Geometry check sheet. Reference: the model listing, model coordinates, mm. Face numbers are marked on the shaded views. Give positions to 0.01 mm unless a question says otherwise; leave off trailing zeros. Loops run counter-clockwise (first coordinate to the right, second up) from the corner with the lowest first, then second, coordinate; pieces in that order, holes last. Notation, with made-up numbers: (0, -38.75) -> (53, -38.75) arc R18 cw to (53, -29.75) -> close; hole circle Ø10 at (7.5, 47). An arc over 180 degrees is marked (long way). One line per question, with ' | ' between items.
from build123d import *

# Parameters (mm, degrees)
F0_R        = 45
F1_DEPTH    = 5
F2_R        = 36
F2_R_2      = 33.5
F3_DEPTH    = 70
F5_DEPTH    = 65
F6_R        = 3.4
F7_DEPTH    = 5.001
F8_T2_ANGLE = 64.3663587264
F8_T4_ANGLE = 60.259047326
F9_SIZE     = 5


# Not quite as in the source:
# - a fillet or chamfer that OpenCascade refuses, or shapes differently, is made with other operations: its cross-section is extruded or revolved along the edge and cut away or added


with BuildPart() as f1:
    # F0 (on Top) → F1 (new body)
    with BuildSketch(Plane.XY):
        Circle(F0_R)
    extrude(amount=F1_DEPTH)

    # F2 (on face) → F3 (join)
    with BuildSketch(Plane.XY.offset(5)):
        Circle(F2_R)
        Circle(F2_R_2, mode=Mode.SUBTRACT)
    extrude(amount=F3_DEPTH)

    # F4 (on face) → F5 (cut)
    with BuildSketch(Plane.XY.offset(75)):
        with BuildLine():
            Line((-23.0004066086, 24.3563399516), (-24.2860665521, 26.5741786595))
            ThreePointArc((-24.2860665521, 26.5741786595), (-34.7900436906, 9.2548830357), (-34.2800852695, -10.9943510002))
            Line((-34.2800852695, -10.9943510002), (-31.8828522812, -10.2826908158))
            ThreePointArc((-31.8828522812, -10.2826908158), (-32.4500946026, 8.321139362), (-23.0004066086, 24.3563399516))
        make_face()
        with BuildLine():
            ThreePointArc((26.9790229265, 23.8355264664), (9.1813045472, 34.8095338494), (-11.7135995274, 34.0410279826))
            Line((-11.7135995274, 34.0410279826), (-10.6344524928, 31.7672538973))
            ThreePointArc((-10.6344524928, 31.7672538973), (8.4559678958, 32.4152218401), (24.7971983706, 22.5244079383))
            Line((24.7971983706, 22.5244079383), (26.9790229265, 23.8355264664))
        make_face()
        with BuildLine():
            ThreePointArc((36, 0), (35.3753586598, 6.6771251068), (33.5231111282, 13.1225386373))
            Line((33.5231111282, 13.1225386373), (31.2720148564, 12.012954958))
            ThreePointArc((31.2720148564, 12.012954958), (32.9382945649, 6.1089075256), (33.5, 0))
            ThreePointArc((33.5, 0), (31.0323255924, -12.619222176), (23.9928496521, -23.3793320173))
            Line((23.9928496521, -23.3793320173), (25.3486350697, -25.562603547))
            ThreePointArc((25.3486350697, -25.562603547), (33.2306399465, -13.8464641243), (36, 0))
        make_face()
        with BuildLine():
            Line((-24.739174036, -22.5881222774), (-26.8374439413, -23.9948244982))
            ThreePointArc((-26.8374439413, -23.9948244982), (-7.1064924362, -35.2916104089), (15.4589834804, -32.5118413775))
            Line((15.4589834804, -32.5118413775), (14.3252158119, -30.2826384574))
            ThreePointArc((14.3252158119, -30.2826384574), (-6.4741042843, -32.8684647301), (-24.739174036, -22.5881222774))
        make_face()
    extrude(amount=-F5_DEPTH, mode=Mode.SUBTRACT)

    # F6 (on face) → F7 (cut, through all)
    with BuildSketch(Plane.XY.offset(5)):
        Circle(F6_R)
    extrude(amount=-F7_DEPTH, mode=Mode.SUBTRACT)

    # F8: chamfer of 5 on 2 edges, made by hand

    # F8_s1 → F8_t2 (revolve, cut)
    with BuildSketch(Plane(origin=(0, 0, 0), x_dir=(0, 0, 1), z_dir=(0.9996677989, -0.0257738601, 0))):
        Polygon((70, -36), (75, -31), (75, -36), align=None)
    revolve(axis=Axis((0, 0, 75), (0, 0, 1)), revolution_arc=F8_T2_ANGLE, mode=Mode.SUBTRACT)

    # F8_s3 → F8_t4 (revolve, cut)
    with BuildSketch(Plane(origin=(0, 0, 0), x_dir=(0, 0, 1), z_dir=(-0.9962472468, -0.0865530086, 0))):
        Polygon((70, -36), (75, -31), (75, -36), align=None)
    revolve(axis=Axis((0, 0, 75), (0, 0, 1)), revolution_arc=F8_T4_ANGLE, mode=Mode.SUBTRACT)

    # F9
    f9_edges = [f1.edges().sort_by_distance(p)[0] for p in [
        (-23.643237, 25.465259, 10),
        (-11.174026, 32.904141, 10),
        (25.888111, 23.179967, 10),
        (32.397563, 12.567747, 10),
        (24.670742, -24.470968, 10),
        (14.8921, -31.39724, 10),
        (-25.788309, -23.291473, 10),
        (-33.081469, -10.638521, 10),
    ]]
    chamfer(f9_edges, length=F9_SIZE)


solid = f1.part
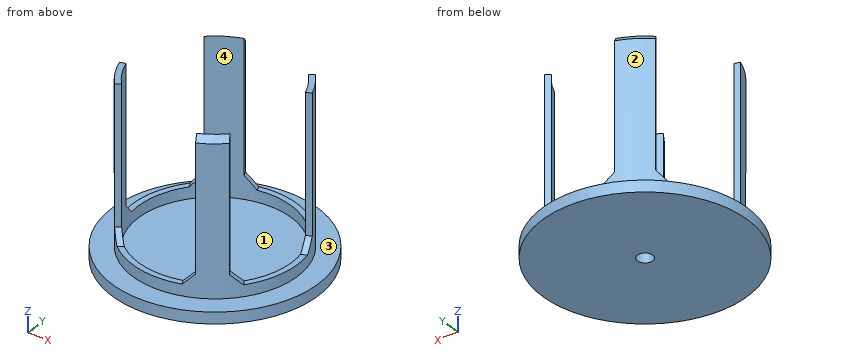
Item 1: Release check for a two-part mould opening along X. For the marked faces 1, 2, 3 and 4 record: pulls with the +X half, pulls with the -X half, needs draft (parallel to the pull), parting line crosses it, or undercut.
Result:
face 1: undercut | face 2: parting line crosses it | face 3: needs draft | face 4: undercut
Item 2: Sectioned sample at C-C (z = 30.5). Record the cut outline in (x, y).
Result:
outline: (-34.28, -10.99) arc R36 ccw to (-26.84, -23.99) -> (-24.74, -22.59) arc R33.5 cw to (-31.88, -10.28) -> close; (-24.29, 26.57) -> (-23, 24.36) arc R33.5 cw to (-10.63, 31.77) -> (-11.71, 34.04) arc R36 ccw to start; (14.33, -30.28) -> (15.46, -32.51) arc R36 ccw to (25.35, -25.56) -> (23.99, -23.38) arc R33.5 cw to start; (24.8, 22.52) arc R33.5 cw to (31.27, 12.01) -> (33.52, 13.12) arc R36 ccw to (26.98, 23.84) -> close
Item 3: Scan lines: probe 1 along Y at (x, z) = (0, 3); probe 2 along Z at (x, y) = (3.5, -3); probe 3 along Z at (x, y) = (-16.5, -30). Record each from-to range of solid material in increasing order.
Result:
probe 1: -45 to -3.4, 3.4 to 45 | probe 2: 0 to 5 | probe 3: 0 to 10
Item 4: Depth check by flat-ended pin: pin 1 Ø5 at (x, z) = (-9.5, 37) entering from +Y; pin 2 Ø7 at (x, y) = (30, -13) entering from +Z; pin 3 Ø10 at (y, z) = (-27, 11.5) entering from +X. Enter the tip coordinate at first touch or a pass-through.
Result:
pin 1: y = 34.04 | pin 2: z = 10 | pin 3: x = 28.43
Item 5: Sectioned sample at A-A (y = 0). Record the cut outline in (x, z).
Result:
outline: (-45, 0) -> (-3.4, 0) -> (-3.4, 5) -> (-33.5, 5) -> (-33.5, 10) -> (-36, 10) -> (-36, 5) -> (-45, 5) -> close; (3.4, 0) -> (45, 0) -> (45, 5) -> (36, 5) -> (36, 10) -> (33.5, 10) -> (33.5, 5) -> (3.4, 5) -> close
